```python
from build123d import *

# Parameters (mm, degrees)
PAD_DEPTH   = 15
FILLET_R    = 1.4
FILLET001_R = 1
FILLET002_R = 1.3


with BuildPart() as part:
    # Sketch → Pad (new body)
    with BuildSketch(Plane.XY):
        Polygon((0, 0), (0, -60), (3, -60), (6, -45.303062), (66, -41.100273), (66, -30.303062), (63, -30.303062), (63, -38.303062), (6, -38.303062), (3, -15.499553), (3, 0), align=None)
    extrude(amount=PAD_DEPTH)

    # Fillet
    fillet_edges = [part.edges().sort_by_distance(p)[0] for p in [
        (34.5, -38.303062, 15),
        (4.5, -26.901307, 15),
        (3, -7.749777, 15),
        (3, -7.749777, 0),
        (4.5, -26.901307, 0),
        (34.5, -38.303062, 0),
        (63, -30.303062, 7.5),
        (66, -30.303062, 7.5),
        (66, -41.100273, 7.5),
        (3, -60, 7.5),
        (3, 0, 7.5),
        (36, -43.201667, 0),
        (36, -43.201667, 15),
    ]]
    fillet(fillet_edges, radius=FILLET_R)

    # Fillet001
    fillet001_edges = [part.edges().sort_by_distance(p)[0] for p in [
        (63, -35.003062, 0),
        (63, -35.003062, 15),
    ]]
    fillet(fillet001_edges, radius=FILLET001_R)

    # Fillet002
    fillet002_edges = [part.edges().sort_by_distance(p)[0] for p in [
        (4.61431, -52.091531, 15),
        (4.61431, -52.091531, 0),
    ]]
    fillet(fillet002_edges, radius=FILLET002_R)


solid = part.part
```
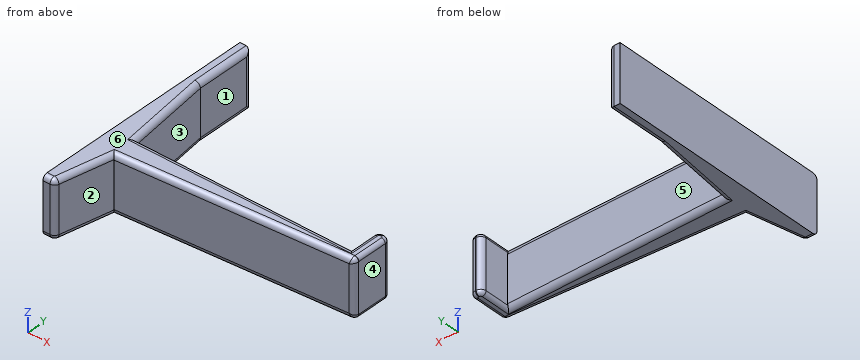
Here's how the part is built. I have some questions about the finished solid (model axes, mm). Face numbers are marked on the shaded views. A direction names the side the tool comes from. Coordinates: 2 decimals unless noted, no trailing zeros. Order: outer loops, then holes, each group sorted by start corner. A loop starts at its lowest first (then second) coordinate and runs counter-clockwise, first axis right, second up. Notation, with made-up numbers: M 47,64.25 L 89,64.25 A23 cw 89,102.25 Z; hole C -5,53 d2. An arc over 180 degrees is marked long. Answer as a JSON object with one key per item and string values. Group by question number.
(1) Suppose I cut it at A-A, the plane z = 12.75. Please give me the cut outline in (x, y), then the cut area to 3 significant figures.
(2) Suppose I cut it at B-B, the plane y = -12. Please give me the cut outline in (x, z).
(3) If we mould it in two halves opening along X, with no side actions, what happens to the marked faces 4, 5 and 6? For each: released by +X, released by -X, zero draft, split by the parting line, or undercut.
(4) Which directions (+Z, -Z, +X, -X, +Y, -Y) give clear straight access to the entire face, cutting with the end or side of a thin tool? Please do the marked faces 1, 2 and 3.
(5) I need wall thicknesses on probe 1 along X at (y, z) = (-8.5, 9.75); probe 2 along X at (y, z) = (-32.5, 4.75); probe 3 along X at (y, z) = (-30.5, 1). Which ranges of each line are inside material? Lowest first, please.
(6) For pin 1 (8 mm diameter, centred on y = -18, z = 5.5, fed in from +X); pin 2 (2 mm diameter, centred on y = -19.5, z = 8, fed in from +X); pin 3 (4 mm diameter, centred on x = 47.5, z = 9, fed in from -Y), each with a flat end and sliding along its axis, tell me the tip position at first contact or that it passes through.
Values found:
{
 "1": {"outline": "M 0,-60 L 1.86,-60 A1.4 ccw 3.23,-58.88 L 6,-45.3 L 64.7,-41.19 A1.4 ccw 66,-39.79 L 66,-31.7 A1.4 ccw 64.6,-30.3 L 64.4,-30.3 A1.4 ccw 63,-31.7 L 63,-38.3 L 6,-38.3 L 3,-15.5 L 3,-1.4 A1.4 ccw 1.6,0 L 0,0 Z", "area": "573 mm^2"},
 "2": {"outline": "M 0,0 L 1.6,0 A1.4 ccw 3,1.4 L 3,13.6 A1.4 ccw 1.6,15 L 0,15 Z"},
 "3": {"face 4": "released by +X", "face 5": "undercut", "face 6": "zero draft"},
 "4": {"face 1": "+Z, -Z, +X, +Y", "face 2": "+Z, -Z, +X, -Y", "face 3": "+Z, -Z, +Y"},
 "5": {"probe 1": "x = 0 to 3", "probe 2": "x = 0 to 5.24, 63 to 66", "probe 3": "x = 0 to 4.91, 63.68 to 65.32"},
 "6": {"pin 1": "stops at x = 3.86", "pin 2": "stops at x = 3.66", "pin 3": "stops at y = -42.54"}
}
